```python
from build123d import *

# Parameters (mm, degrees)
SCHIZZO1_R                   = 7.5
ESTRUSIONE_ESTRUSIONE1_DEPTH = 1.5
ESTRUSIONE_ESTRUSIONE2_START = 9
ESTRUSIONE_ESTRUSIONE2_DEPTH = 9


with BuildPart() as part:
    # Schizzo1 → Estrusione-Estrusione1 (new body)
    with BuildSketch(Plane.XY):
        with BuildLine():
            Line((17.05, -17.5), (0, -17.5))
            ThreePointArc((0, -17.5), (-17.5, 0), (0, 17.5))
            Line((0, 17.5), (17.05, 17.5))
            Line((17.05, 17.5), (17.05, -17.5))
        make_face()
        Circle(SCHIZZO1_R, mode=Mode.SUBTRACT)
    extrude(amount=ESTRUSIONE_ESTRUSIONE1_DEPTH)

    # Schizzo2 → Estrusione-Estrusione2 (add)
    with BuildSketch(Plane(origin=(0, 0, 0), x_dir=(-1, 0, 0), z_dir=(0, 0, -1)).offset(ESTRUSIONE_ESTRUSIONE2_START)):
        with BuildLine():
            Line((-17.05, 17.5), (0, 17.5))
            ThreePointArc((0, 17.5), (17.5, 0), (0, -17.5))
            Line((0, -17.5), (-17.05, -17.5))
            Line((-17.05, -17.5), (-17.05, -16.5))
            Line((-17.05, -16.5), (0, -16.5))
            ThreePointArc((0, -16.5), (16.5, 0), (0, 16.5))
            Line((0, 16.5), (-17.05, 16.5))
            Line((-17.05, 16.5), (-17.05, 17.5))
        make_face()
    extrude(amount=-ESTRUSIONE_ESTRUSIONE2_DEPTH)


solid = part.part
```
Check sheet for the modelled part. Datum: model origin and axes. Units: mm. A direction names the side the tool comes from. Round coordinates to 2 decimals unless told otherwise and drop trailing zeros. Order: outer loops, then holes, each group sorted by start corner. A loop starts at its lowest first (then second) coordinate and runs counter-clockwise, first axis right, second up. Notation, with made-up numbers: M -29,-9.75 L -16,-9.75 A15 cw -16,16.25 Z; hole C 75,62.25 d5. An arc over 180 degrees is marked long. Answer in a Markdown table with one row per item.
(1) Draft check along Y on faces 1 (the cylindrical face through (-16.496, -0.363, -4.563)), 2 (the flat face through (-16, 5, -9)), 3 (the flat face through (8, -17.5, -4)). Enter one of: +Y half, -Y half, draft (parallel to the pull), parting line (faces both ways), or undercut.
Findings:
| item | result |
|---|---|
| face 1 | undercut |
| face 2 | draft |
| face 3 | -Y half |
(2) Gauge pin test, flat ends, axial feed: pin 1 (4 mm diameter, centred on y = -11, z = -3, fed in from -X); pin 2 (5 mm diameter, centred on x = 4.5, y = -4.5, fed in from -Z); pin 3 (3 mm diameter, centred on x = -5.5, z = -5, fed in from +Y). Record the tip position at first contact, or that the pin passes through.
Findings:
| item | result |
|---|---|
| pin 1 | stops at x = -15.01 |
| pin 2 | stops at z = 0 |
| pin 3 | stops at y = 17.04 |
(3) Set-up check for faces 4 (the flat face through (9, -16.5, -5)), 5 (the flat face through (8, 0, 1.5)): record each of +Z, -Z, +X, -X, +Y, -Y from which the full face is reachable in a straight line by a thin tool's end or side.
Findings:
| item | result |
|---|---|
| face 4 | -Z, +X |
| face 5 | +Z, +X, -X, +Y, -Y |
(4) Section check D-D on x = 8.5. Record the boundary of the cut face in (y, z), plus the area to 3 significant figures.
Findings:
| item | result |
|---|---|
| outline | M -17.5,-9 L -16.5,-9 L -16.5,0 L 16.5,0 L 16.5,-9 L 17.5,-9 L 17.5,1.5 L -17.5,1.5 Z |
| area | 70.5 mm^2 |
(5) Section check C-C on z = -5. Record the boundary of the cut face in (x, y), plus the area to 3 significant figures.
Findings:
| item | result |
|---|---|
| outline | M 0,-17.5 L 17.05,-17.5 L 17.05,-16.5 L 0,-16.5 A16.5 cw 0,16.5 L 17.05,16.5 L 17.05,17.5 L 0,17.5 A17.5 ccw Z |
| area | 87.5 mm^2 |
(6) Section check B-B on x = -5. Record the boundary of the cut face in (y, z).
Findings:
| item | result |
|---|---|
| outline | M -16.77,-9 L -15.72,-9 L -15.72,0 L -5.59,0 L -5.59,1.5 L -16.77,1.5 Z; M 5.59,0 L 15.72,0 L 15.72,-9 L 16.77,-9 L 16.77,1.5 L 5.59,1.5 Z |
(7) Section check A-A on y = 0. Record the boundary of the cut face in (x, z), plus the area to 3 significant figures.
Findings:
| item | result |
|---|---|
| outline | M -17.5,-9 L -16.5,-9 L -16.5,0 L -7.5,0 L -7.5,1.5 L -17.5,1.5 Z; M 7.5,0 L 17.05,0 L 17.05,1.5 L 7.5,1.5 Z |
| area | 38.3 mm^2 |
(8) Material ranges on line 1 along Y through (x, z) = (0, 0.85); line 2 along Y through (x, z) = (14, -1.5); line 3 along Z through (x, y) = (-4.5, 10), recorded low to high. Write a range as from..to.
Findings:
| item | result |
|---|---|
| line 1 | y = -17.5..-7.5, 7.5..17.5 |
| line 2 | y = -17.5..-16.5, 16.5..17.5 |
| line 3 | z = 0..1.5 |
